from build123d import *

# Parameters (mm, degrees)
SKETCH1_W           = 23
SKETCH1_H           = 12
BOSS_EXTRUDE1_DEPTH = 32
CUT_EXTRUDE1_DEPTH  = 7.5
SKETCH3_R           = 6
SKETCH3_R_2         = 2.4
CUT_EXTRUDE2_DEPTH  = 3.5
SKETCH4_W           = 32
SKETCH4_H           = 12
SKETCH4_R           = 1.25
BOSS_EXTRUDE2_DEPTH = 2.4


with BuildPart() as part:
    # Sketch1 → Boss-Extrude1 (new body)
    with BuildSketch(Plane.XY):
        with Locations((11.5, 6)):
            Rectangle(SKETCH1_W, SKETCH1_H)
    extrude(amount=BOSS_EXTRUDE1_DEPTH)

    # Sketch2 → Cut-Extrude1 (cut)
    with BuildSketch(Plane.XY.offset(32)):
        with BuildLine():
            Line((17, 12), (0, 12))
            Line((0, 12), (0, 0))
            Line((0, 0), (17, 0))
            ThreePointArc((17, 0), (11, 6), (17, 12))
        make_face()
        with BuildLine():
            Line((23, 12), (17, 12))
            ThreePointArc((17, 12), (21.242640687, 10.242640687), (23, 6))
            Line((23, 6), (23, 12))
        make_face()
        with BuildLine():
            ThreePointArc((23, 6), (21.242640687, 1.757359313), (17, 0))
            Line((17, 0), (23, 0))
            Line((23, 0), (23, 6))
        make_face()
    extrude(amount=-CUT_EXTRUDE1_DEPTH, mode=Mode.SUBTRACT)

    # Sketch3 → Cut-Extrude2 (cut)
    with BuildSketch(Plane.XY.offset(32)):
        with Locations((17, 6)):
            Circle(SKETCH3_R)
        with Locations((17, 6)):
            Circle(SKETCH3_R_2, mode=Mode.SUBTRACT)
    extrude(amount=-CUT_EXTRUDE2_DEPTH, mode=Mode.SUBTRACT)

    # Sketch4 → Boss-Extrude2 (add)
    with BuildSketch(Plane.XY.offset(19.5)):
        with Locations((11.5, 6)):
            Rectangle(SKETCH4_W, SKETCH4_H)
        with Locations((24.65, 6)):
            Circle(SKETCH4_R, mode=Mode.SUBTRACT)
        with Locations((-1.65, 6)):
            Circle(SKETCH4_R, mode=Mode.SUBTRACT)
    extrude(amount=BOSS_EXTRUDE2_DEPTH)


solid = part.part
Source: CAD feature listing. Evaluate the final solid. Frame: model axes, mm. A direction names the side the tool comes from. Give positions to 0.01 mm unless a question says otherwise; leave off trailing zeros. Loops run counter-clockwise (first coordinate to the right, second up) from the corner with the lowest first, then second, coordinate; pieces in that order, holes last. Notation, with made-up numbers: (40.25, 76.5) -> (44.25, 76.5) arc R23 cw to (44.25, 100.5) -> close; hole circle Ø8 at (-16, -24.75). An arc over 180 degrees is marked (long way). Use a Markdown table: item, result. Add a question column.
1) Section query C-C, the plane y = 10.25. Return the cut outline in (x, z), then the cut area to 3 significant figures.
2) Pull-direction query (Y, two-part tool) for faces 1 (the face through (23, 6, 10)), 2 (the face through (24.38, 4.78, 20.68)), 3 (the face through (11, 0, 12)); classes: +Y half, -Y half, draft (parallel to the pull), parting line (faces both ways), or undercut.
3) First-contact query: pin 1 (5 mm diameter, centred on x = 19.5, y = 4, fed in from +Z); pin 2 (3 mm diameter, centred on y = 6.5, z = 23.5, fed in from +X); pin 3 (3.5 mm diameter, centred on y = 8, z = 12.5, fed in from -X); pin 4 (1.3 mm diameter, centred on x = 26, y = 4.5, fed in from +Z). Flat tips, straight axial feed; report the tip coordinate or a pass-through.
4) Section query B-B, the plane y = 6.5. Count the separate pieces of the cut face and the enclosed holes in it, then the cut area to 3 significant figures.
5) Reachability of faces 4 (the face through (0, 6, 10)), 5 (the face through (14.602, 6.106, 30.274)), 6 (the face through (0, 6, 23)), 7 (the face through (26.2, 6.1, 19.5)), 8 (the face through (23, 6, 23)) from +Z, -Z, +X, -X, +Y, -Y: full face, straight path, thin tool, end or side. Return the list, or none.
6) Section query A-A, the plane x = -1.65. Return the cut outline in (y, z).
7) Line query: line 1 along Y through (x, z) = (-1.65, 20.3); line 2 along X through (y, z) = (7, 18); line 3 along Z through (x, y) = (4.5, 2.5). Output: solid intervals per line, ascending. Write a range as [from, to].
8) Section query D-D, the plane z = 25.5. Return the cut outline in (x, y).
Numbers:
| question | item | result |
|---|---|---|
| 1 | outline | (-4.5, 19.5) -> (0, 19.5) -> (0, 0) -> (23, 0) -> (23, 19.5) -> (27.5, 19.5) -> (27.5, 21.9) -> (23, 21.9) -> (23, 24.5) -> (21.24, 24.5) -> (21.24, 28.5) -> (12.76, 28.5) -> (12.76, 24.5) -> (0, 24.5) -> (0, 21.9) -> (-4.5, 21.9) -> close |
| 1 | area | 619 mm2 |
| 2 | face 1 | draft |
| 2 | face 2 | undercut |
| 2 | face 3 | -Y half |
| 3 | pin 1 | stops at z = 32 |
| 3 | pin 2 | stops at x = 23 |
| 3 | pin 3 | stops at x = 0 |
| 3 | pin 4 | stops at z = 21.9 |
| 4 | separate pieces | 3 |
| 4 | enclosed holes | 0 |
| 4 | area | 638 mm2 |
| 5 | face 4 | -Z, -X, +Y, -Y |
| 5 | face 5 | +Z |
| 5 | face 6 | +Z, -X, +Y, -Y |
| 5 | face 7 | -Z, +X, +Y, -Y |
| 5 | face 8 | +Z, +X, +Y, -Y |
| 6 | outline | (0, 19.5) -> (4.75, 19.5) -> (4.75, 21.9) -> (0, 21.9) -> close; (7.25, 19.5) -> (12, 19.5) -> (12, 21.9) -> (7.25, 21.9) -> close |
| 7 | line 1 | y = [0, 4.75], [7.25, 12] |
| 7 | line 2 | x = [0, 23] |
| 7 | line 3 | z = [0, 24.5] |
| 8 | outline | circle Ø12 at (17, 6) |
